The listing builds one solid part. Answer for the finished solid, in the listing's coordinates (mm). A direction names the side the tool comes from. Round coordinates to 2 decimals unless told otherwise and drop trailing zeros. Order: outer loops, then holes, each group sorted by start corner. A loop starts at its lowest first (then second) coordinate and runs counter-clockwise, first axis right, second up. Notation, with made-up numbers: (42.25, 83) - (53.25, 83) arc R7 cw to (53.25, 93) - close; hole circle Ø6 at (58, -12). An arc over 180 degrees is marked (long way). Use CSV: the item, a comma, the result in double quotes. Start each with the question number.
Item 1: Find section A-A, the plane x = 0. Give the vertices of the cut face in (y, z) (3 decimals).
Item 2: Find section C-C, the plane z = 12.5. Give the vertices of the cut face in (x, y), plus the area to 3 significant figures.
Item 3: Find section B-B, the plane z = 15.5. Give the vertices of the cut face in (x, y), plus the area to 3 significant figures.
Item 4: Determine the mould class of faces 1 (the flat face through (-0.202, -9.694, 19.465)), 2 (the flat face through (0, 0, 8.4)), 3 (the cylindrical face through (5.08, -0.177, 16.426)) for opening direction Y: +Y half, -Y half, draft (parallel to the pull), parting line (faces both ways), or undercut.
Item 5: Flat-ended cylindrical pins translate along their axes: P1, Ø1.5, axis at x = -8, z = 3.5, coming from the -Y side; P2, Ø2, axis at x = -7.5, z = 6, coming from the -Y side; P3, Ø10, axis at x = 9, z = 2.5, coming from the -Y side (3 decimals). Find the tip coordinate at first contact, or state that the pin passes through.
Item 6: For faces 4 (the flat face through (0, -12.159, 16)), 5 (the flat face through (-3.922, 0, 21)), 6 (the flat face through (0, 2.111, 4)), 7 (the flat face through (3.577, 0, 21)), 8 (the flat face through (0, 12.052, 16)), determine the directions among +Z, -Z, +X, -X, +Y, -Y from which every point of the face is accessible in a straight line to the end or side of a thin tool.
Item 7: Straight lines are drawn through the part: line 1 along X through (y, z) = (0, 6.25) (3 decimals); line 2 along Y through (x, z) = (0, 6) (3 decimals); line 3 along Z through (x, y) = (1.75, 0). For each, find the intervals that lie inside material, in ascending order. Write a range as [from, to].
```python
from build123d import *

# Parameters (mm, degrees)
F0_R         = 12.625
F0_R_2       = 10.375
F0_R_3       = 5
F1_DEPTH     = 15
F2_DEPTH     = 15
F3_R         = 12.6739646699
F4_DEPTH     = 6.6
F6_DEPTH     = 7
F7_T4_DEPTH  = 36.6039255786
F7_S5_R      = 12.6739646699
F7_T6_DEPTH  = 20
F7_T10_DEPTH = 24.210816556
F7_S11_R     = 12.6739646699
F7_T12_DEPTH = 14
F8_T1_DEPTH  = 32.8699146781
F9_T1_DEPTH  = 33.2150521969
F10_R        = 5


# Not quite as in the source:
# - a fillet or chamfer that OpenCascade refuses, or shapes differently, is made with other operations: its cross-section is extruded or revolved along the edge and cut away or added
# - a feature names something its author has since deleted; it is built from what else it names


with BuildPart() as f1:
    # F0 (on Top) → F1 (new body)
    with BuildSketch(Plane.XY):
        Circle(F0_R)
        Circle(F0_R_2, mode=Mode.SUBTRACT)
        Circle(F0_R_2)
        Circle(F0_R_3, mode=Mode.SUBTRACT)
    extrude(amount=F1_DEPTH)

    # F0 (on Top) → F2 (join)
    with BuildSketch(Plane.XY):
        Circle(F0_R_3)
        with BuildLine():
            ThreePointArc((2.304625, 2.1105280404), (2.9126944678, 1.1321819366), (3.125, 0))
            ThreePointArc((3.125, 0), (-1.1321819366, -2.9126944678), (-2.304625, 2.1105280404))
            ThreePointArc((-2.304625, 2.1105280404), (0, 3.125), (2.304625, 2.1105280404))
        make_face(mode=Mode.SUBTRACT)
        with BuildLine():
            Line((-2.304625, 2.1105280404), (2.304625, 2.1105280404))
            ThreePointArc((2.304625, 2.1105280404), (0, 3.125), (-2.304625, 2.1105280404))
        make_face()
    extrude(amount=F2_DEPTH)

    # F3 (on face) → F4 (join)
    with BuildSketch(Plane.XY.offset(15)):
        Circle(F3_R)
    extrude(amount=-F4_DEPTH)

    # F5 (on face) → F6 (join)
    with BuildSketch(Plane.XY.offset(15)):
        with BuildLine():
            Line((3.5765423992, 12.0519627893), (-3.921679918, 12.0519627893))
            Line((-3.921679918, 12.0519627893), (-3.921679918, -12.0519627893))
            ThreePointArc((-3.921679918, -12.0519627893), (-3.7494920856, -12.1066382433), (-3.5765423992, -12.1588537667))
            Line((-3.5765423992, -12.1588537667), (3.5765423992, -12.1588537667))
            Line((3.5765423992, -12.1588537667), (3.5765423992, 12.0519627893))
        make_face()
    extrude(amount=F6_DEPTH)

    # F7: fillet of radius 5 on 2 edges, made by hand


with BuildPart() as f7_tool2:
    # F7_s3 → F7_t4 (new body)
    with BuildSketch(Plane.XZ.offset(-12.0519627893)):
        with BuildLine():
            ThreePointArc((-8.921679918, 15), (-5.3861460121, 16.4644660941), (-3.921679918, 20))
            Line((-3.921679918, 20), (-3.921679918, 15))
            Line((-3.921679918, 15), (-8.921679918, 15))
        make_face()
    extrude(amount=F7_T4_DEPTH)

    # F7_s5 → F7_t6 (intersect, symmetric)
    with BuildSketch(Plane.XY.offset(17.5)):
        Circle(F7_S5_R)
    extrude(amount=F7_T6_DEPTH, both=True, mode=Mode.INTERSECT)


with BuildPart() as f1_1:
    add(f1.part)

    # F7_t1: union F7_tool2
    add(f7_tool2.part)


with BuildPart() as f7_tool8:
    # F7_s9 → F7_t10 (new body)
    with BuildSketch(Plane.XZ.offset(12.1588537667)):
        with BuildLine():
            ThreePointArc((8.5765423992, 15), (5.0410084933, 16.4644660941), (3.5765423992, 20))
            Line((3.5765423992, 20), (3.5765423992, 15))
            Line((3.5765423992, 15), (8.5765423992, 15))
        make_face()
    extrude(amount=-F7_T10_DEPTH)

    # F7_s11 → F7_t12 (intersect, symmetric)
    with BuildSketch(Plane.XY.offset(17.5)):
        Circle(F7_S11_R)
    extrude(amount=F7_T12_DEPTH, both=True, mode=Mode.INTERSECT)


with BuildPart() as f1_2:
    add(f1_1.part)

    # F7_t7: union F7_tool8
    add(f7_tool8.part)

    # F8: chamfer of 5 on 1 edges, made by hand

    # F8_s2 → F8_t1 (cut)
    with BuildSketch(Plane.YZ.offset(-16.434957339)):
        Polygon((-12.1588537667, 17), (-7.1588537667, 22), (-12.1588537667, 22), align=None)
    extrude(amount=F8_T1_DEPTH, mode=Mode.SUBTRACT)

    # F9: chamfer of 5 on 1 edges, made by hand

    # F9_s2 → F9_t1 (cut)
    with BuildSketch(Plane.YZ.offset(-16.7800948578)):
        Polygon((12.0519627893, 17), (7.0519627893, 22), (12.0519627893, 22), align=None)
    extrude(amount=F9_T1_DEPTH, mode=Mode.SUBTRACT)

    # F10
    f10_edges = [f1_2.edges().sort_by_distance(p)[0] for p in [
        (-12.625, 0, 0),
    ]]
    fillet(f10_edges, radius=F10_R)


solid = f1_2.part
```
Worked out:
1,outline,"(-12.674, 8.4) - (-12.625, 8.4) - (-12.625, 5) arc R5 ccw to (-7.625, 0) - (-3.125, 0) - (-3.125, 8.4) - (2.111, 8.4) - (2.111, 0) - (7.625, 0) arc R5 ccw to (12.625, 5) - (12.625, 8.4) - (12.674, 8.4) - (12.674, 15) - (12.052, 15) - (12.052, 17) - (7.052, 22) - (-7.159, 22) - (-12.159, 17) - (-12.159, 15) - (-12.674, 15) - close"
2,outline,"circle Ø25.35 at (0, 0)"
2,area,"505 mm²"
3,outline,"(-6.74, -10.73) arc R12.67 ccw to (-3.58, -12.16) - (3.58, -12.16) arc R12.67 ccw to (6.4, -10.94) - (6.4, 10.94) arc R12.67 ccw to (3.92, 12.05) - (-3.92, 12.05) arc R12.67 ccw to (-6.74, 10.73) - close"
3,area,"312 mm²"
4,face 1,"-Y half"
4,face 2,"undercut"
4,face 3,"draft"
5,P1,"stops at y = -10.11"
5,P2,"stops at y = -10.82"
5,P3,"stops at y = -11.805"
6,face 4,"+Z, +X, -X, -Y"
6,face 5,"+Z, -X, +Y, -Y"
6,face 6,"-Z"
6,face 7,"+Z, +X, +Y, -Y"
6,face 8,"+Z, +X, -X, +Y"
7,line 1,"x = [-12.625, -3.125], [3.125, 12.625]"
7,line 2,"y = [-12.625, -3.125], [2.111, 12.625]"
7,line 3,"z = [8.4, 22]"
